from build123d import *

# Parameters (mm, degrees)
SKETCH1_W           = 35
SKETCH1_H           = 35
BOSS_EXTRUDE1_DEPTH = 2.5
SKETCH2_W           = 5
SKETCH2_H           = 35
BOSS_EXTRUDE2_DEPTH = 50
SKETCH5_W           = 17
SKETCH5_H           = 35
CUT_EXTRUDE2_DEPTH  = 4
SKETCH6_W           = 30
SKETCH6_H           = 10
BOSS_EXTRUDE3_DEPTH = 16
SKETCH7_W           = 28
SKETCH7_H           = 13.5
CUT_EXTRUDE3_DEPTH  = 16


with BuildPart() as part:
    # Sketch1 → Boss-Extrude1 (new body)
    with BuildSketch(Plane(origin=(0, 0, 0), x_dir=(1, 0, 0), z_dir=(0, 1, 0))):
        with Locations((17.5, 17.5)):
            Rectangle(SKETCH1_W, SKETCH1_H)
    extrude(amount=BOSS_EXTRUDE1_DEPTH)

    # Sketch2 → Boss-Extrude2 (add)
    with BuildSketch(Plane(origin=(0, 2.5, 0), x_dir=(1, 0, 0), z_dir=(0, 1, 0))):
        with Locations((2.5, 17.5)):
            Rectangle(SKETCH2_W, SKETCH2_H)
    extrude(amount=BOSS_EXTRUDE2_DEPTH)

    # Sketch5 → Cut-Extrude2 (cut)
    with BuildSketch(Plane.ZY):
        with Locations((-17.553851225, 30)):
            Rectangle(SKETCH5_W, SKETCH5_H)
    extrude(amount=-CUT_EXTRUDE2_DEPTH, mode=Mode.SUBTRACT)

    # Sketch6 → Boss-Extrude3 (add)
    with BuildSketch(Plane(origin=(0, 2.5, 0), x_dir=(1, 0, 0), z_dir=(0, 1, 0))):
        with Locations((20, 5)):
            Rectangle(SKETCH6_W, SKETCH6_H)
    extrude(amount=BOSS_EXTRUDE3_DEPTH)

    # Sketch7 → Cut-Extrude3 (cut)
    with BuildSketch(Plane.XY):
        with Locations((19, 9.3)):
            Rectangle(SKETCH7_W, SKETCH7_H)
    extrude(amount=-CUT_EXTRUDE3_DEPTH, mode=Mode.SUBTRACT)


solid = part.part
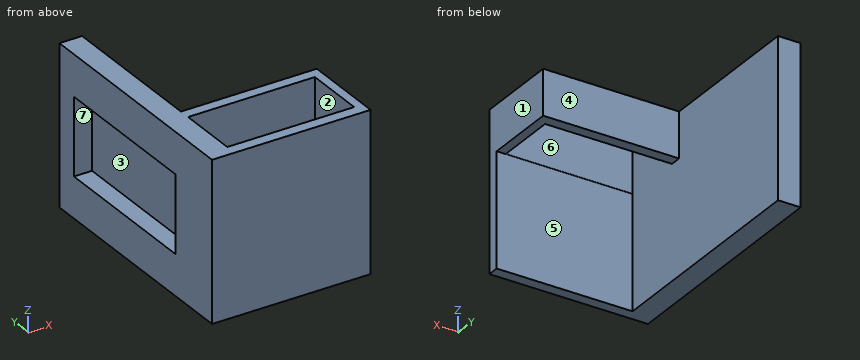
Verification items for the finished model (mm, model axes). Face numbers are marked on the shaded views. A direction names the side the tool comes from. Coordinates: 2 decimals unless noted, no trailing zeros. Loops run counter-clockwise (first coordinate to the right, second up) from the corner with the lowest first, then second, coordinate; pieces in that order, holes last. Notation, with made-up numbers: (84, -10) -> (123, -10) arc R21 ccw to (123, 1) -> close; hole circle Ø3 at (20, 4). An arc over 180 degrees is marked (long way). Answer as a JSON object with one key per item and string values. Group by question number.
Item 1: Scan lines: probe 1 along Y at (x, z) = (2.5, -11); probe 2 along Y at (x, z) = (7, -6); probe 3 along X at (y, z) = (10.5, -2). Record each from-to range of solid material in increasing order.
Item 2: Sectioned sample at B-B on y = 6.5. Record the boundary of the cut face in (x, z), plus the area to 3 significant figures.
Item 3: Mould release check, pull along X, two halves, no side actions. Record for the marked faces 1, 2 and 3: +X half, -X half, draft (parallel to the pull), parting line (faces both ways), or undercut.
Item 4: Sectioned sample at A-A on x = 20. Record the boundary of the cut face in (y, z).
Item 5: Depth check by flat-ended pin: pin 1 (6 mm diameter, centred on y = 41.5, z = -14.5, fed in from +X); pin 2 (12.5 mm diameter, centred on x = 21.5, z = -17.5, fed in from +Y); pin 3 (3 mm diameter, centred on x = 13, z = -7, fed in from +Y). Enter the tip coordinate at first touch or a pass-through.
Item 6: Sectioned sample at D-D on x = 3. Record the boundary of the cut face in (y, z).
Item 7: Sectioned sample at C-C on z = -4. Record the boundary of the cut face in (x, y).
Item 8: Tool access check on the marked faces 4, 5, 6 and 7. Record the directions out of +Z, -Z, +X, -X, +Y, -Y that give a thin tool (end or side, any length) a straight path to the whole face; none if there is none.
Evaluation:
{
 "1": {"probe 1": "y = 0 to 12.5, 47.5 to 52.5", "probe 2": "y = 0 to 2.55, 16.05 to 18.5", "probe 3": "x = 0 to 5, 33 to 35"},
 "2": {"outline": "(0, -35) -> (5, -35) -> (5, 0) -> (0, 0) -> close; (33, -10) -> (35, -10) -> (35, 0) -> (33, 0) -> close", "area": "195 mm²"},
 "3": {"face 1": "+X half", "face 2": "undercut", "face 3": "-X half"},
 "4": {"outline": "(0, -35) -> (2.5, -35) -> (2.5, -10) -> (2.55, -10) -> (2.55, 0) -> (0, 0) -> close; (16.05, -10) -> (18.5, -10) -> (18.5, 0) -> (16.05, 0) -> close"},
 "5": {"pin 1": "stops at x = 5", "pin 2": "stops at y = 2.5", "pin 3": "stops at y = 18.5"},
 "6": {"outline": "(0, -35) -> (52.5, -35) -> (52.5, 0) -> (0, 0) -> close; hole (12.5, -26.05) -> (47.5, -26.05) -> (47.5, -9.05) -> (12.5, -9.05) -> close"},
 "7": {"outline": "(0, 0) -> (35, 0) -> (35, 18.5) -> (5, 18.5) -> (5, 52.5) -> (0, 52.5) -> close; hole (5, 2.55) -> (33, 2.55) -> (33, 16.05) -> (5, 16.05) -> close"},
 "8": {"face 4": "+Z, -Z, +X, +Y", "face 5": "-Z, +X, +Y", "face 6": "+Z, -Z", "face 7": "-X"}
}
